Here's how the part is built. I have some questions about the finished solid (model axes, mm). A direction names the side the tool comes from. Coordinates: 2 decimals unless noted, no trailing zeros. Loops run counter-clockwise (first coordinate to the right, second up) from the corner with the lowest first, then second, coordinate; pieces in that order, holes last. Notation, with made-up numbers: (-18, -29) -> (16, -29) arc R9 cw to (16, -18) -> close; hole circle Ø3 at (60, 74.5). An arc over 180 degrees is marked (long way). Use CSV: the item, a comma, the result in double quotes. Start each with the question number.
from build123d import *

# Parameters (mm, degrees)
F2_DEPTH = 12
F3_DEPTH = 6
F4_R     = 1.6
F5_DEPTH = 25


with BuildPart() as f2:
    # F1 (on Top) → F2 (new body)
    with BuildSketch(Plane.XY):
        with BuildLine():
            Line((8, 0), (6.2, 0))
            ThreePointArc((6.2, 0), (4.384062, -4.384062), (0, -6.2))
            Line((0, -6.2), (0, -8))
            ThreePointArc((0, -8), (5.656854, -5.656854), (8, 0))
        make_face()
        with BuildLine():
            Line((26, 0), (8, 0))
            ThreePointArc((8, 0), (5.656854, -5.656854), (0, -8))
            Line((0, -8), (0, -12))
            Line((0, -12), (26, -12))
            Line((26, -12), (26, 0))
        make_face()
        with BuildLine():
            Line((0, -8), (0, -6.2))
            ThreePointArc((0, -6.2), (-4.384062, -4.384062), (-6.2, 0))
            Line((-6.2, 0), (-8, 0))
            ThreePointArc((-8, 0), (-5.656854, -5.656854), (0, -8))
        make_face()
        with BuildLine():
            Line((0, -12), (0, -8))
            ThreePointArc((0, -8), (-5.656854, -5.656854), (-8, 0))
            Line((-8, 0), (-26, 0))
            Line((-26, 0), (-26, -12))
            Line((-26, -12), (0, -12))
        make_face()
    extrude(amount=F2_DEPTH)

    # F1 (on Top) → F3 (cut)
    with BuildSketch(Plane.XY):
        with BuildLine():
            Line((0, -8), (0, -6.2))
            ThreePointArc((0, -6.2), (-4.384062, -4.384062), (-6.2, 0))
            Line((-6.2, 0), (-8, 0))
            ThreePointArc((-8, 0), (-5.656854, -5.656854), (0, -8))
        make_face()
        with BuildLine():
            Line((8, 0), (6.2, 0))
            ThreePointArc((6.2, 0), (4.384062, -4.384062), (0, -6.2))
            Line((0, -6.2), (0, -8))
            ThreePointArc((0, -8), (5.656854, -5.656854), (8, 0))
        make_face()
    extrude(amount=F3_DEPTH, mode=Mode.SUBTRACT)

    # F4 (on face) → F5 (cut)
    with BuildSketch(Plane.XZ.offset(12)):
        with Locations((-21.3, 6)):
            Circle(F4_R)
        with Locations((21.3, 6)):
            Circle(F4_R)
    extrude(amount=-F5_DEPTH, mode=Mode.SUBTRACT)


solid = f2.part
1) Thinking about a two-plate mould opening in X: for faces 3 (the face through (-26, -6, 6)), 4 (the face through (0, -7, 12)), 5 (the face through (-19.82, -6.08, 5.39)), which applies, pulls with the +X half, pulls with the -X half, needs draft (parallel to the pull), parting line crosses it, or undercut?
2) I want a section at D-D, the plane x = -1. Please give me the cut outline in (y, z).
3) Please list where these lines run through material, in increasing order: L1, parallel to Z at x = -21.3, y = -4; L2, parallel to Z at x = 7, y = -3.5; L3, parallel to X at y = -7.25, z = 0.5. Write a range as [from, to].
4) I want a section at C-C, the plane z = 8.25. Please give me the cut outline in (x, y), plus the area to 3 significant figures.
5) I want a section at A-A, the plane y = -2.5. Please give me the cut outline in (x, z).
6) Which directions (+Z, -Z, +X, -X, +Y, -Y) give clear straight access to the entire face, cutting with the end or side of a thin tool? Please do faces 1 (the face through (0, -6.4, 6)), 2 (the face through (19.7, -6.08, 6.07)).
7) I want a section at B-B, the plane x = -21.3. Please give me the cut outline in (y, z).
Return value:
1,face 3,"pulls with the -X half"
1,face 4,"needs draft"
1,face 5,"undercut"
2,outline,"(-12, 0) -> (-7.94, 0) -> (-7.94, 6) -> (-6.12, 6) -> (-6.12, 12) -> (-12, 12) -> close"
3,L1,"z = [0, 4.4], [7.6, 12]"
3,L2,"z = [6, 12]"
3,L3,"x = [-26, -3.38], [3.38, 26]"
4,outline,"(-26, -12) -> (26, -12) -> (26, 0) -> (6.2, 0) arc R6.2 cw to (-6.2, 0) -> (-26, 0) -> close"
4,area,"564 mm²"
5,outline,"(-26, 0) -> (-7.6, 0) -> (-7.6, 6) -> (-5.67, 6) -> (-5.67, 12) -> (-26, 12) -> close; (5.67, 6) -> (7.6, 6) -> (7.6, 0) -> (26, 0) -> (26, 12) -> (5.67, 12) -> close; hole circle Ø3.2 at (-21.3, 6); hole circle Ø3.2 at (21.3, 6)"
6,face 1,"-Z, +Y"
6,face 2,"+Y, -Y"
7,outline,"(-12, 0) -> (0, 0) -> (0, 4.4) -> (-12, 4.4) -> close; (-12, 7.6) -> (0, 7.6) -> (0, 12) -> (-12, 12) -> close"
